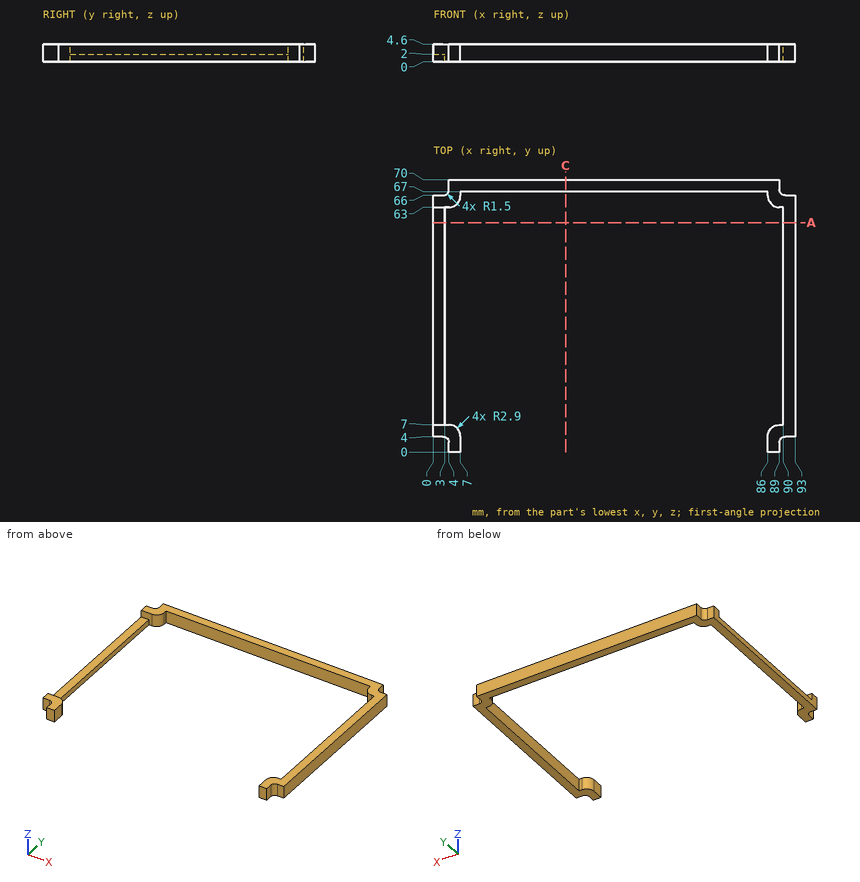
Check sheet for the drawn part. Datum: minimum x, y, z corner. Units: mm. Round coordinates to 2 decimals unless told otherwise and drop trailing zeros. Order: outer loops, then holes, each group sorted by start corner. A loop starts at its lowest first (then second) coordinate and runs counter-clockwise, first axis right, second up.
(1) Cross-section at C-C, the plane x = 34. Enter the section's corners in (y, z), and give its area (3 significant figures).
(2) Scan lines: probe 1 along X at (y, z) = (28.5, 1.2); probe 2 along Y at (x, z) = (71, 3.45); probe 3 along X at (y, z) = (46.5, 3.25). Record each from-to range of solid material in increasing order.
(3) Go/stop test with flat-tipped pins: P1, Ø2, axis at x = 91.5, z = 2.5, coming from the -Y side; P2, Ø1.2, axis at y = 66.5, z = 3, coming from the +X side; P3, Ø1, axis at x = 13.5, z = 3, coming from the -Y side; P4, Ø1.2, axis at y = 2, z = 2, coming from the +X side. Record where each tip stops, or that it passes through.
(4) Cross-section at A-A, the plane y = 59. Enter the section's corners in (x, z).
Check sheet entries:
1. outline: (67, 0) - (70, 0) - (70, 4.6) - (67, 4.6) - close
1. area: 13.8 mm2
2. probe 1: x = 0 to 3, 90 to 93
2. probe 2: y = 67 to 70
2. probe 3: x = 90 to 93
3. P1: stops at y = 4
3. P2: stops at x = 93
3. P3: stops at y = 67
3. P4: stops at x = 89
4. outline: (0, 0) - (3, 0) - (3, 2) - (0, 2) - close; (90, 0) - (93, 0) - (93, 4.6) - (90, 4.6) - close
